from build123d import *

# Parameters (mm, degrees)
F0_W      = 1200
F0_H      = 600
F1_DEPTH  = 340
F2_W      = 400
F2_H      = 54.2701794954
F3_DEPTH  = 600
F4_W      = 700
F4_H      = 400
F5_DEPTH  = 160
F6_R      = 80
F7_DEPTH  = 500.001
F9_DEPTH  = 150
F10_R     = 60
F11_DEPTH = 150


with BuildPart() as f1:
    # F0 (on Top) → F1 (new body)
    with BuildSketch(Plane.XY):
        Rectangle(F0_W, F0_H)
    extrude(amount=F1_DEPTH)

    # F2 (on face) → F3 (cut)
    with BuildSketch(Plane.XZ.offset(300)):
        with Locations((0, 312.8649102523)):
            Rectangle(F2_W, F2_H)
    extrude(amount=-F3_DEPTH, mode=Mode.SUBTRACT)

    # F4 (on face) → F5 (join)
    with BuildSketch(Plane(origin=(0, 0, 0), x_dir=(1, 0, 0), z_dir=(0, 0, -1))):
        Rectangle(F4_W, F4_H)
    extrude(amount=F5_DEPTH)

    # F6 (on face) → F7 (cut, through all)
    with BuildSketch(Plane(origin=(0, 0, -160), x_dir=(1, 0, 0), z_dir=(0, 0, -1))):
        Circle(F6_R)
    extrude(amount=-F7_DEPTH, mode=Mode.SUBTRACT)

    # F8 (on face) → F9 (cut)
    with BuildSketch(Plane(origin=(0, 0, 0), x_dir=(1, 0, 0), z_dir=(0, 0, -1))):
        with BuildLine():
            Line((600, -150), (600, 150))
            ThreePointArc((600, 150), (450, 0), (600, -150))
        make_face()
    extrude(amount=-F9_DEPTH, mode=Mode.SUBTRACT)

    # F10
    f10_edges = [f1.edges().sort_by_distance(p)[0] for p in [
        (-350, 200, -80),
        (350, 200, -80),
        (350, -200, -80),
        (-350, -200, -80),
    ]]
    fillet(f10_edges, radius=F10_R)

    # F8 (on face) → F11 (cut)
    with BuildSketch(Plane(origin=(0, 0, 0), x_dir=(1, 0, 0), z_dir=(0, 0, -1))):
        with BuildLine():
            ThreePointArc((-600, -120.9617067128), (-493.933982822, -77.0277238908), (-450, 29.0382932872))
            ThreePointArc((-450, 29.0382932872), (-493.933982822, 135.1043104651), (-600, 179.0382932872))
            Line((-600, 179.0382932872), (-600, -120.9617067128))
        make_face()
    extrude(amount=-F11_DEPTH, mode=Mode.SUBTRACT)


solid = f1.part
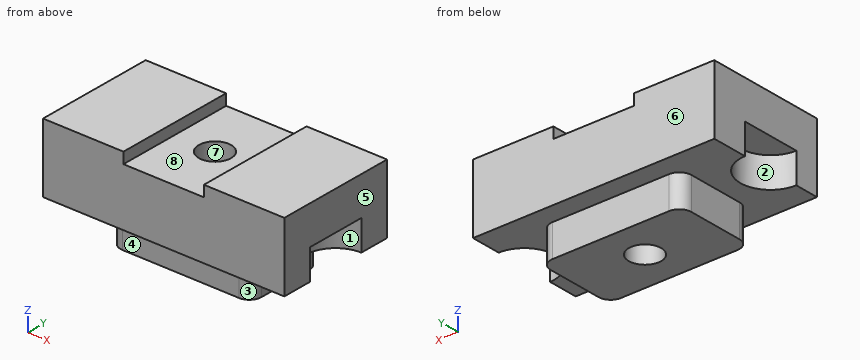
Model file for the job. Use its own axes, mm. Face numbers are marked on the shaded views. A direction names the side the tool comes from. Give positions to 0.01 mm unless a question says otherwise; leave off trailing zeros. Loops run counter-clockwise (first coordinate to the right, second up) from the corner with the lowest first, then second, coordinate; pieces in that order, holes last.
Item 1: Slice it at C-C (z = 116). Write the cut outline in (x, y).
Check values:
outline: (-600, -300) - (600, -300) - (600, -150) arc R150 cw to (600, 150) - (600, 300) - (-600, 300) - (-600, 120.96) arc R150 cw to (-600, -179.04) - close; hole circle Ø160 at (0, 0)
Item 2: Slice it at D-D (y = -214). Write the cut outline in (x, z), plus the area to 3 significant figures.
Check values:
outline: (-600, 0) - (600, 0) - (600, 340) - (200, 340) - (200, 285.73) - (-200, 285.73) - (-200, 340) - (-600, 340) - close
area: 386,000 mm2
Item 3: Slice it at A-A (x = 0). Write the cut outline in (y, z), plus the area to 3 significant figures.
Check values:
outline: (-300, 0) - (-200, 0) - (-200, -160) - (-80, -160) - (-80, 285.73) - (-300, 285.73) - close; (80, -160) - (200, -160) - (200, 0) - (300, 0) - (300, 285.73) - (80, 285.73) - close
area: 164,000 mm2
Item 4: Mould opens along X. For the marked faces 5, 6, 7 and 8 say: +X half, -X half, draft (parallel to the pull), parting line (faces both ways), or undercut.
Check values:
face 5: +X half
face 6: draft
face 7: undercut
face 8: undercut
Item 5: Which spindle directions (+Z, -Z, +X, -X, +Y, -Y) get a long thin tool onto all of the face, cutting with end or side? Do the marked faces 1, 2, 3 and 4. Say none if no direction does.
Check values:
face 1: -Z, +X
face 2: -Z, -X
face 3: -Z, +X, -Y
face 4: -Z, +X, -X, -Y
Item 6: Slice it at B-B (y = -21). Write the cut outline in (x, z).
Check values:
outline: (-600, 150) - (-450.22, 150) - (-450.22, 0) - (-350, 0) - (-350, -160) - (-77.19, -160) - (-77.19, 285.73) - (-200, 285.73) - (-200, 340) - (-600, 340) - close; (77.19, -160) - (350, -160) - (350, 0) - (451.48, 0) - (451.48, 150) - (600, 150) - (600, 340) - (200, 340) - (200, 285.73) - (77.19, 285.73) - close
Item 7: Drill centre lines: line 1 along Y through (x, z) = (0, -31); line 2 along X through (y, z) = (0, 177); line 3 along Y through (x, z) = (0, 81). Where is each one in solid material? Low to high.
Check values:
line 1: y = -200 to -80, 80 to 200
line 2: x = -600 to -80, 80 to 600
line 3: y = -300 to -80, 80 to 300
Item 8: Drop flat-ended pins along their axis: P1, Ø6, axis at x = 67, z = -1.5, coming from the +Y side; P2, Ø4, axis at y = 179.5, z = -49.5, coming from the -X side; P3, Ø3, axis at y = 101.5, z = -28.5, coming from the -X side; P4, Ø6, axis at x = 157.5, y = 90, coming from the +Z side. Give the stop position or say it passes through.
Check values:
P1: stops at y = 300
P2: stops at x = -336.84
P3: stops at x = -350
P4: stops at z = 285.73
